```python
from build123d import *

# Parameters (mm, degrees)
SKETCH2_W           = 250
SKETCH2_H           = 200
BOSS_EXTRUDE1_DEPTH = 25
FILLET1_R           = 10
FILLET2_R           = 10
FILLET3_R           = 10
FILLET4_R           = 10
SKETCH3_R           = 1.6
CUT_EXTRUDE1_DEPTH  = 26
SKETCH4_R           = 22.5
CUT_EXTRUDE2_DEPTH  = 26


with BuildPart() as part:
    # Sketch2 → Boss-Extrude1 (new body)
    with BuildSketch(Plane(origin=(0, 0, 0), x_dir=(1, 0, 0), z_dir=(0, 1, 0))):
        with Locations((125, 100)):
            Rectangle(SKETCH2_W, SKETCH2_H)
    extrude(amount=BOSS_EXTRUDE1_DEPTH)

    # Fillet1
    fillet1_edges = [part.edges().sort_by_distance(p)[0] for p in [
        (0, 12.5, 0),
    ]]
    fillet(fillet1_edges, radius=FILLET1_R)

    # Fillet2
    fillet2_edges = [part.edges().sort_by_distance(p)[0] for p in [
        (250, 12.5, 0),
    ]]
    fillet(fillet2_edges, radius=FILLET2_R)

    # Fillet3
    fillet3_edges = [part.edges().sort_by_distance(p)[0] for p in [
        (250, 12.5, -200),
    ]]
    fillet(fillet3_edges, radius=FILLET3_R)

    # Fillet4
    fillet4_edges = [part.edges().sort_by_distance(p)[0] for p in [
        (0, 12.5, -200),
    ]]
    fillet(fillet4_edges, radius=FILLET4_R)

    # Sketch3 → Cut-Extrude1 (cut, through all)
    with BuildSketch(Plane(origin=(0, 25, 0), x_dir=(1, 0, 0), z_dir=(0, 1, 0))):
        with Locations((84.183925072, 129.712061316)):
            Circle(SKETCH3_R)
        with Locations((82.913925072, 81.676079735)):
            Circle(SKETCH3_R)
        with Locations((165.463925072, 81.676079735)):
            Circle(SKETCH3_R)
        with Locations((159.113925072, 129.712061316)):
            Circle(SKETCH3_R)
        with Locations((134.983925072, 86.756079735)):
            Circle(SKETCH3_R)
    extrude(amount=-CUT_EXTRUDE1_DEPTH, mode=Mode.SUBTRACT)

    # Sketch4 → Cut-Extrude2 (cut, through all)
    with BuildSketch(Plane(origin=(0, 25, 0), x_dir=(1, 0, 0), z_dir=(0, 1, 0))):
        with Locations((203.930975459, 168.75038786)):
            Circle(SKETCH4_R)
        with Locations((203.930975459, 34.26608254)):
            Circle(SKETCH4_R)
        with Locations((39.910397475, 34.26608254)):
            Circle(SKETCH4_R)
        with Locations((39.910397475, 168.75038786)):
            Circle(SKETCH4_R)
    extrude(amount=-CUT_EXTRUDE2_DEPTH, mode=Mode.SUBTRACT)


solid = part.part
```
Read the model definition and answer for the solid it produces. Units are mm, in the model's axes. Give positions to 0.01 mm unless a question says otherwise; leave off trailing zeros. Order: outer loops, then holes, each group sorted by start corner. A loop starts at its lowest first (then second) coordinate and runs counter-clockwise, first axis right, second up. Notation, with made-up numbers: (79.25, 89) -> (96.25, 89) arc R17 ccw to (96.25, 114) -> close; hole circle Ø2 at (70.5, -3). An arc over 180 degrees is marked (long way). Write item = value, one per line.
1. A cutting plane is placed at C-C, the plane y = 20.5. Count the separate pieces of the cut face and the enclosed holes in it, and give its area (3 significant figures).
Numbers:
separate_pieces = 1
enclosed_holes = 9
area = 43,500 mm²
2. The mould has two halves that part along Z. Classify faces 1 (the face through (2.85, 12.68, -3.01)), 2 (the face through (0, 12, -99)), 3 (the face through (181.453, 12.675, -35.255)): +Z half, -Z half, draft (parallel to the pull), parting line (faces both ways), or undercut.
Numbers:
face_1 = +Z half
face_2 = draft
face_3 = undercut
3. A cutting plane is placed at B-B, the plane x = 56. Write down the section's boundary in (y, z), and give its area (3 significant figures).
Numbers:
outline = (0, -200) -> (25, -200) -> (25, -184.48) -> (0, -184.48) -> close; (0, -153.02) -> (25, -153.02) -> (25, -49.99) -> (0, -49.99) -> close; (0, -18.54) -> (25, -18.54) -> (25, 0) -> (0, 0) -> close
area = 3,430 mm²
4. Straight lines are drawn through the part: line 1 along Z through (x, y) = (41.5, 9.5); line 2 along Z through (x, y) = (208, 18.5); line 3 along X through (y, z) = (19.5, -44). For each, find the intervals that lie inside material, in ascending order.
Numbers:
line_1 = -200 to -191.19, -146.31 to -56.71, -11.82 to 0
line_2 = -200 to -190.88, -146.62 to -56.4, -12.14 to 0
line_3 = 0 to 19.62, 60.2 to 183.65, 224.22 to 250
5. A cutting plane is placed at A-A, the plane z = -41. Write down the section's boundary in (x, y).
Numbers:
outline = (0, 0) -> (18.44, 0) -> (18.44, 25) -> (0, 25) -> close; (61.38, 0) -> (182.46, 0) -> (182.46, 25) -> (61.38, 25) -> close; (225.4, 0) -> (250, 0) -> (250, 25) -> (225.4, 25) -> close
